Geometry check sheet. Reference: the model listing, model coordinates, mm. Face numbers are marked on the shaded views. A direction names the side the tool comes from. Coordinates: 2 decimals unless noted, no trailing zeros. Order: outer loops, then holes, each group sorted by start corner. A loop starts at its lowest first (then second) coordinate and runs counter-clockwise, first axis right, second up. Notation, with made-up numbers: M -15,10.5 L 30,10.5 A31 ccw 30,40.5 Z; hole C -38,47 d6. An arc over 180 degrees is marked long. One line per item, written item: value. Start each with the question number.
1) Draft check along Z on the marked faces 1, 2, 3 and 4. Enter one of: pulls with the +Z half, pulls with the -Z half, needs draft (parallel to the pull), parting line crosses it, or undercut.
2) Sectioned sample at D-D, the plane y = 10. State how many separate pieces and enclosed holes the cut face has, then the cut area to 3 significant figures.
3) Sectioned sample at A-A, the plane x = 19.5. Enter the section's corners in (y, z), then the cut area to 3 significant figures.
4) Access from +Z, -Z, +X, -X, +Y, -Y to the whole of each face (thin tool, end or side, straight path). Record for the marked faces 5, 6 and 7.
5) Thickness scan on L1, parallel to X at y = 1, z = 3; L2, parallel to X at y = -12, z = -10.5 (3 decimals); L3, parallel to X at y = -13, z = 0.5. Record the ranges inside material, lowest first. Write a range as from..to.
6) Sectioned sample at B-B, the plane y = -7.5. Enter the section's corners in (x, z) (3 decimals).
7) Go/stop test with flat-tipped pins: P1, Ø11, axis at x = 24, y = -12, coming from the -Z side; P2, Ø1, axis at y = -10.5, z = -12, coming from the +X side; P3, Ø4.5, axis at x = 21, y = -9, coming from the +Z side. Record where each tip stops, or that it passes through.
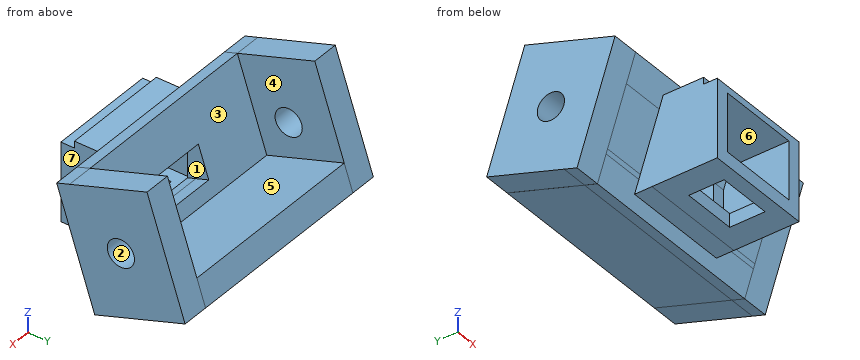
Autodesk Inventor part; units mm, degrees
ref_plane "Work Plane1" through (0, -6.818, 6.8414) normal (0, -1, 0) x (1, 0, 0)
ref_plane "YZ Plane" through (0, 0, 0) normal (1, 0, 0) x (0, 1, 0)
ref_plane "XZ Plane" through (0, 0, 0) normal (0, 1, 0) x (-1, 0, 0)
sketch "Sketch8" plane through (0, 0, 0) normal (1, 0, 0) x (0, 1, 0)
  line L0 (-3.8078, 7.851) -> (3.0591, -12.6251)
  line L1 (-0.2897, -12.6251) -> (-4.6863, 0.485)
  line L2 (3.0591, -12.6251) -> (-0.2897, -12.6251)
  line L3 (-4.6863, 0.485) -> (-6.818, 6.8414)
  line L4 (-3.8078, 7.851) -> (-6.818, 6.8414)
  point P0 (0, 0)
extrude "Extrusion6" add sketch "Sketch8" along normal blind 45.72
sketch "Sketch11" plane through (0, 0, 0) normal (-1, 0, 0) x (0, 0, 1)
  line L0 (0.485, -4.6863) -> (-12.6251, -0.2897)
  line L1 (7.851, -6.8159) -> (0.485, -6.8159)
  line L2 (7.851, -6.8159) -> (0.485, -6.8159)
  line L3 (0.485, -6.8159) -> (0.485, -4.6863)
  line L4 (-12.6251, -0.2897) -> (0.485, -4.6863)
  line L5 (7.851, -3.8078) -> (-12.6251, 3.0591)
  line L6 (0.485, -6.8159) -> (7.851, -6.8159)
  line L7 (13.9082, 14.2533) -> (7.851, -3.808)
  line L8 (7.851, -3.808) -> (-18.639, 5.076)
  line L9 (-18.639, 5.076) -> (-12.5817, 23.1373)
  line L10 (-12.5817, 23.1373) -> (13.9082, 14.2533)
  point P0 (0, 0)
  dimension "d73" = 27.94
  dimension "d74" = 18.54
  dimension "d76" = 0
  dimension "d88" = 19.05
extrude "Extrusion8" add sketch "Sketch11" along normal blind 6.35
sketch "Sketch13" plane through (0, -3.8078, 7.851) normal (0, 0.9481042, 0.3179598) x (1, 0, 0)
  line L0 (0, 0) -> (0, 21.5968)
  line L1 (16.51, 18.0408) -> (29.21, 18.0408)
  line L2 (29.21, 18.0408) -> (29.21, 10.4208)
  line L3 (29.21, 10.4208) -> (16.51, 10.4208)
  line L4 (16.51, 10.4208) -> (16.51, 18.0408)
  point P0 (0, 8.6543)
  dimension "d55" = 7.62
  dimension "d56" = 12.7
  dimension "d57" = 16.51
extrude "Extrusion10" cut sketch "Sketch13" against normal blind 25.4
sketch "Sketch15" plane through (0, 0, 0) normal (1, 0, 0) x (0, 0, -1)
  line L0 (-0.485, -6.8159) -> (-7.851, -6.8159)
  line L1 (6.5678, 21.1205) -> (12.5883, 23.1395)
  line L2 (12.5883, 23.1395) -> (18.6455, 5.0782)
  line L3 (18.6455, 5.0782) -> (12.6251, 3.0591)
  line L4 (12.6251, 3.0591) -> (6.5678, 21.1205)
  dimension "d67" = 6.35
  dimension "d68" = 18.54
  dimension "d69" = 0
  dimension "d70" = 0
  dimension "d87" = 19.05
extrude "Extrusion11" add sketch "Sketch15" along normal blind 45.72
sketch "Sketch17" plane through (45.72, 0, 0) normal (1, 0, 0) x (0, 0, -1)
  line L0 (-7.851, -3.808) -> (-13.9082, 14.2533)
  line L1 (-7.851, -3.808) -> (-13.9082, 14.2533)
  line L2 (-13.9082, 14.2533) -> (12.5883, 23.1395)
  line L3 (12.5883, 23.1395) -> (18.6456, 5.0782)
  line L4 (18.6456, 5.0782) -> (-7.851, -3.808)
  point P0 (0, 0)
extrude "Extrusion12" add sketch "Sketch17" along normal blind 6.35
sketch "Sketch19" plane through (45.72, 5.0782, -18.6456) normal (0, -0.9481019, -0.3179666) x (1, 0, 0)
  line L0 (0, 6.3501) -> (0, 0.0001)
  line L1 (6.35, 27.947) -> (0, 27.947)
  line L2 (0, 27.947) -> (0, 0.0001)
  line L3 (0, 0.0001) -> (6.35, 0.0001)
  line L4 (6.35, 0.0001) -> (6.35, 27.947)
  line L5 (-45.72, 6.3501) -> (0, 6.3501)
  line L6 (0, 0.0001) -> (0, 0.0001)
  line L7 (0, 0.0001) -> (0, 6.3501)
  line L8 (0, 6.3501) -> (0, 6.3501)
  line L9 (0, 6.3501) -> (0, 0.0001)
  line L10 (-45.72, 0.007) -> (-52.07, 0.007)
  line L11 (-52.07, 0.007) -> (-45.72, 0.007)
  line L12 (-45.72, 0.007) -> (-45.72, 27.947)
  line L13 (-45.72, 27.947) -> (-52.07, 27.947)
  line L14 (-52.07, 27.947) -> (-52.07, 0.007)
  point P0 (-45.72, 19.2926)
extrude "Extrusion13" add sketch "Sketch19" along normal blind 3.175
sketch "Sketch20" plane through (0, 5.0782, -18.6455) normal (0, -0.9481019, -0.3179666) x (1, 0, 0)
  line L0 (45.72, 0) -> (0, 0)
  line L1 (0, 0) -> (0, 6.35)
  line L2 (0, 6.35) -> (45.72, 6.35)
  line L3 (45.72, 6.35) -> (45.72, 0)
  point P0 (0, 19.2926)
extrude "Extrusion14" add sketch "Sketch20" along normal blind 3.175
sketch "Sketch21" plane through (0, 0, 0) normal (1, 0, 0) x (0, 0, -1)
  line L0 (19.6485, 2.0658) -> (13.6346, 0.0489)
  line L1 (13.6346, 0.0489) -> (12.6251, 3.0591)
  line L2 (12.6251, 3.0591) -> (12.6251, -0.2897)
  line L3 (12.6251, -0.2897) -> (-6.8414, -6.818)
  line L4 (-0.485, -4.6863) -> (-0.485, -4.6865)
  line L5 (19.6485, 2.0657) -> (-6.8414, -6.8182)
  line L6 (19.6485, 2.0657) -> (19.6485, 2.0658)
  line L7 (12.6251, 3.0591) -> (13.6346, 0.0489)
  line L8 (12.6251, -0.2897) -> (13.6346, 0.0489)
  line L9 (12.6251, 3.0591) -> (12.6251, -0.2897)
  point P0 (0, 0)
  point P1 (-6.8415, -6.8181)
extrude "Extrusion15" add sketch "Sketch21" along normal blind 45.72
sketch "Sketch22" plane through (16.51, -1.0818, -10.2631) normal (0, 0.9481042, 0.3179598) x (1, 0, 0)
  line L0 (12.7, -7.62) -> (12.7, 0)
  line L1 (12.7, 0) -> (0, 0)
  line L2 (0, 0) -> (12.7, 0)
  line L3 (12.7, 0) -> (12.7, -7.62)
  line L4 (12.7, -7.62) -> (0, -7.62)
  line L5 (0, -7.62) -> (0, 0)
  point P0 (-16.51, -9.3866)
extrude "Extrusion16" cut sketch "Sketch22" against normal blind 45.72
sketch "Sketch23" plane through (52.07, 0, 0) normal (1, 0, 0) x (0, 0, -1)
  circle A0 centre (2.8734, 8.1606) radius 3.175
  point P0 (0, 0)
  dimension "d89" = 6.35
extrude "Extrusion17" cut sketch "Sketch23" against normal blind 76.2
ref_plane "Work Plane1" through (0, -6.818, 6.8414) normal (0, -1, 0) x (1, 0, 0)
sketch "Sketch25" plane through (0, -6.818, 6.8414) normal (0, -1, 0) x (1, 0, 0)
  line L0 (35.56, -20.2796) -> (35.56, -3.5301)
  line L1 (35.56, -3.5301) -> (32.385, -3.5301)
  line L2 (32.385, -3.5301) -> (32.385, -20.2796)
  line L3 (32.385, -6.7051) -> (10.16, -6.7051)
  line L4 (10.16, -6.7051) -> (10.16, -3.5301)
  line L5 (10.16, -3.5301) -> (32.385, -3.5301)
  line L6 (32.385, -3.5301) -> (32.385, -6.7051)
  line L7 (10.16, -6.7051) -> (13.335, -6.7051)
  line L8 (13.335, -6.7051) -> (13.335, -20.2796)
  line L9 (10.16, -20.2796) -> (10.16, -6.7051)
  line L10 (13.335, -20.2796) -> (32.385, -20.2796)
  line L11 (32.385, -20.2796) -> (32.385, -23.4546)
  line L12 (32.385, -23.4546) -> (13.335, -23.4546)
  line L13 (13.335, -23.4546) -> (13.335, -20.2796)
  line L14 (29.21, -17.1046) -> (16.51, -17.1046)
  line L15 (29.21, -9.8801) -> (29.21, -17.1046)
  line L16 (16.51, -9.8801) -> (29.21, -9.8801)
  line L17 (16.51, -17.1046) -> (16.51, -9.8801)
  line L18 (32.385, -23.4546) -> (35.56, -23.4546)
  line L19 (35.56, -23.4546) -> (35.56, -3.5301)
  line L20 (35.56, -3.5301) -> (32.385, -3.5301)
  line L21 (32.385, -3.5301) -> (32.385, -23.4546)
  line L22 (32.385, -3.5301) -> (10.16, -3.5301)
  line L23 (10.16, -3.5301) -> (10.16, -6.7051)
  line L24 (10.16, -6.7051) -> (32.385, -6.7051)
  line L25 (32.385, -6.7051) -> (32.385, -3.5301)
  line L26 (10.16, -6.7051) -> (13.335, -6.7051)
  line L27 (13.335, -6.7051) -> (13.335, -23.4546)
  line L28 (13.335, -23.4546) -> (10.16, -23.4546)
  line L29 (10.16, -23.4546) -> (10.16, -6.7051)
  line L30 (32.385, -20.2796) -> (13.335, -20.2796)
  line L31 (13.335, -20.2796) -> (13.335, -23.4546)
  line L32 (13.335, -23.4546) -> (32.385, -23.4546)
  line L33 (32.385, -23.4546) -> (32.385, -20.2796)
  line L34 (35.56, -3.5301) -> (32.385, -3.5301)
  line L35 (32.385, -3.5301) -> (32.385, -23.4546)
  line L36 (32.385, -23.4546) -> (35.56, -23.4546)
  line L37 (35.56, -23.4546) -> (35.56, -3.5301)
  point P0 (0, -6.8414)
  dimension "d102" = 3.175
  dimension "d103" = 3.175
  dimension "d104" = 3.175
  dimension "d105" = 3.175
  dimension "d106" = 3.175
  dimension "d107" = 3.175
  dimension "d108" = 3.175
  dimension "d109" = 3.175
extrude "Extrusion18" add sketch "Sketch25" against normal blind 3.81 contours L19 L18 L11 L2 L1 L0 | L2 L3 L4 L5 | L12 L13 L10 L11 | L28 L29 L9 L3 L8 L13
sketch "Sketch26" plane through (35.56, -6.818, 3.3114) normal (1, 0, 0) x (0, 0, -1)
  line L0 (7.8311, 3.81) -> (19.9245, 3.81)
  line L1 (7.8311, 3.81) -> (19.9245, 3.81)
  line L2 (19.9245, 3.81) -> (19.9245, 7.8658)
  line L3 (19.9245, 7.8658) -> (7.8311, 3.81)
  point P0 (3.3114, 6.818)
extrude "Extrusion19" add sketch "Sketch26" against normal blind 25.4
sketch "Sketch27" plane through (16.51, -1.0818, -10.2632) normal (0, 0.9481013, 0.3179684) x (1, 0, 0)
  line L0 (0, -6.0578) -> (12.7, -6.0578)
  line L1 (12.7, -6.0578) -> (12.7, 0)
  line L2 (12.7, 0) -> (0, 0)
  line L3 (0, 0) -> (0, -6.0578)
  point P0 (-16.51, -9.3865)
extrude "Extrusion20" cut sketch "Sketch27" against normal blind 25.4
sketch "Sketch28" plane through (0, -6.818, 6.8414) normal (0, -1, 0) x (1, 0, 0)
  line L0 (10.16, -3.5301) -> (10.16, -23.4546)
  line L1 (35.56, -23.4546) -> (35.56, -3.5301)
  line L2 (35.56, -3.5301) -> (10.16, -3.5301)
  line L3 (32.385, -6.7051) -> (13.335, -6.7051)
  line L4 (32.385, -6.7051) -> (32.385, -20.2796)
  line L5 (32.385, -20.2796) -> (13.335, -20.2796)
  line L6 (13.335, -20.2796) -> (13.335, -6.7051)
  line L7 (35.56, -23.4546) -> (29.21, -23.4546)
  line L8 (29.21, -23.4546) -> (29.21, -20.2796)
  line L9 (29.21, -20.2796) -> (35.56, -20.2796)
  line L10 (35.56, -20.2796) -> (35.56, -23.4546)
  line L11 (10.16, -23.4546) -> (16.51, -23.4546)
  line L12 (16.51, -23.4546) -> (16.51, -20.2796)
  line L13 (16.51, -20.2796) -> (10.16, -20.2796)
  line L14 (10.16, -20.2796) -> (10.16, -23.4546)
  line L15 (13.335, -6.7051) -> (13.335, -11.3612)
  line L16 (10.16, -20.2796) -> (13.335, -20.2796)
  line L17 (13.335, -20.2796) -> (13.335, -6.7051)
  line L18 (13.335, -6.7051) -> (10.16, -6.7051)
  line L19 (10.16, -6.7051) -> (10.16, -20.2796)
  line L20 (10.16, -3.5301) -> (35.56, -3.5301)
  line L21 (10.16, -6.7051) -> (35.56, -6.7051)
  line L22 (35.56, -6.7051) -> (35.56, -3.5301)
  line L23 (35.56, -3.5301) -> (10.16, -3.5301)
  line L24 (10.16, -3.5301) -> (10.16, -6.7051)
  line L25 (35.56, -6.7051) -> (32.385, -6.7051)
  line L26 (32.385, -6.7051) -> (32.385, -20.2796)
  line L27 (32.385, -20.2796) -> (35.56, -20.2796)
  line L28 (35.56, -20.2796) -> (35.56, -6.7051)
  point P0 (0, -6.8414)
  dimension "d116" = 6.35
  dimension "d117" = 6.35
extrude "Extrusion21" add sketch "Sketch28" along normal blind 8.255 contours L2 L1 L21 L3 L18 L0 | L18 L6 L13 L0 | L13 L5 L12 L11 L0 | L1 L9 L4 L21 | L1 L7 L8 L5 L9
sketch "Sketch29" plane through (0, -15.073, 6.8414) normal (0, -1, 0) x (1, 0, 0)
  line L0 (35.56, -6.3565) -> (35.56, -23.4546)
  line L1 (10.16, -23.4546) -> (35.56, -23.4546)
  line L2 (35.56, -23.4546) -> (35.56, -20.2796)
  line L3 (35.56, -20.2796) -> (10.16, -20.2796)
  line L4 (10.16, -20.2796) -> (10.16, -23.4546)
  line L5 (10.16, -23.4546) -> (10.16, -6.3565)
  line L6 (10.16, -6.7051) -> (35.56, -6.7051)
  line L7 (35.56, -6.7051) -> (32.385, -6.7051)
  line L8 (32.385, -6.7051) -> (32.385, -20.2796)
  line L9 (32.385, -20.2796) -> (35.56, -20.2796)
  line L10 (35.56, -20.2796) -> (35.56, -6.7051)
  line L11 (13.335, -6.7051) -> (10.16, -6.7051)
  line L12 (10.16, -6.7051) -> (10.16, -20.2796)
  line L13 (10.16, -20.2796) -> (13.335, -20.2796)
  line L14 (13.335, -20.2796) -> (13.335, -6.7051)
  line L15 (10.16, -6.3565) -> (10.16, -3.5301)
  line L16 (35.56, -6.7051) -> (10.16, -6.7051)
  line L17 (10.16, -6.7051) -> (10.16, -5.1176)
  line L18 (10.16, -5.1176) -> (35.56, -5.1176)
  line L19 (35.56, -5.1176) -> (35.56, -6.7051)
  point P0 (35.56, -3.5301)
  point P1 (0, -6.8414)
  dimension "d124" = 1.5875
extrude "Extrusion22" add sketch "Sketch29" along normal blind 3.175 contours L0 L6 L5 L15 L18 L19 | L0 L3 L8 L6 | L0 L1 L4 L3 | L14 L3 L5 L6
equation "\"d57\" = d58"
properties part number "Lidar Sensor Case v2"
Final values:
1. face 1: undercut
1. face 2: undercut
1. face 3: pulls with the +Z half
1. face 4: needs draft
2. separate pieces: 3
2. enclosed holes: 0
2. area: 615 mm^2
3. outline: M -18.25,-16.61 L -15.07,-16.61 L -15.07,-13.44 L -18.25,-13.44 Z; M -18.25,0.14 L -4.57,0.14 L -3.5,-3.04 L -0.49,-2.03 L -3.81,7.85 L -6.82,6.84 L -5.63,3.31 L -15.07,3.31 L -15.07,1.72 L -18.25,1.72 Z; M -6.82,-16.61 L 1.05,-16.61 L 2.07,-19.66 L 5.08,-18.65 L 23.14,-12.59 L 21.12,-6.57 L 3.06,-12.63 L 1.93,-9.25 L -1.08,-10.26 L -3.01,-10.91 L -3.01,-13.44 L -6.82,-13.44 Z
3. area: 263 mm^2
4. face 5: +Z
4. face 6: -Y
4. face 7: -Z, +X, -Y
5. L1: x = -6.35..0, 45.72..52.07
5. L2: x = 10.16..13.335, 32.385..35.56
5. L3: x = 10.16..35.56
6. outline: M 10.16,-16.613 L 16.51,-16.613 L 16.51,-13.438 L 13.335,-13.438 L 13.335,0.136 L 32.385,0.136 L 32.385,-13.438 L 29.21,-13.438 L 29.21,-16.613 L 35.56,-16.613 L 35.56,3.311 L 10.16,3.311 Z
7. P1: stops at z = -16.61
7. P2: stops at x = 35.56
7. P3: stops at z = 6.86
